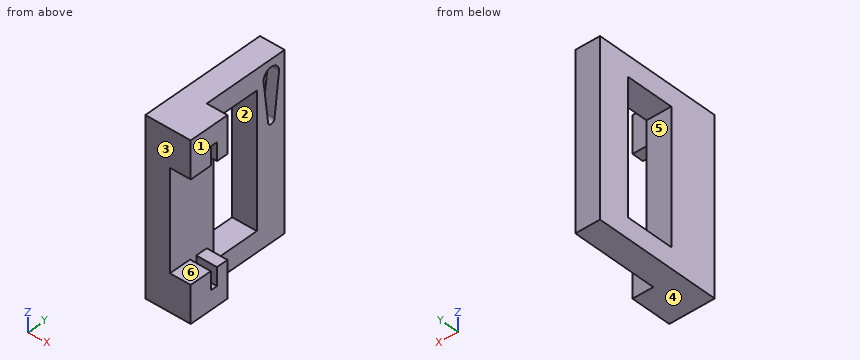
from build123d import *

# Parameters (mm, degrees)
BOSS_EXTRUDE1_DEPTH = 9
SKETCH2_W           = 8.4
SKETCH2_H           = 40.5
CUT_EXTRUDE1_DEPTH  = 40.4
SKETCH3_W           = 18.4
SKETCH3_H           = 70.5
BOSS_EXTRUDE2_DEPTH = 42.5
CUT_EXTRUDE2_DEPTH  = 8.4
SKETCH5_W           = 70.5
SKETCH5_H           = 35
CUT_EXTRUDE3_DEPTH  = 8.4
CUT_EXTRUDE4_DEPTH  = 4.6
SKETCH8_W           = 54
SKETCH8_H           = 19.4972
CUT_EXTRUDE5_DEPTH  = 11


with BuildPart() as part:
    # Sketch1 → Boss-Extrude1 (new body)
    with BuildSketch(Plane(origin=(0, 0, 0), x_dir=(1, 0, 0), z_dir=(0, 1, 0))):
        Polygon((8.4, -15), (8.4, 0), (8.4, 40.5), (8.4, 55.5), (-10, 55.5), (-10, -15), align=None)
    extrude(amount=BOSS_EXTRUDE1_DEPTH)

    # Sketch2 → Cut-Extrude1 (cut)
    with BuildSketch(Plane(origin=(0, 9, 0), x_dir=(1, 0, 0), z_dir=(0, 1, 0))):
        with Locations((4.2, 20.25)):
            Rectangle(SKETCH2_W, SKETCH2_H)
    extrude(amount=-CUT_EXTRUDE1_DEPTH, mode=Mode.SUBTRACT)

    # Sketch3 → Boss-Extrude2 (add)
    with BuildSketch(Plane(origin=(0, 9, 0), x_dir=(1, 0, 0), z_dir=(0, 1, 0))):
        with Locations((-0.8, 20.25)):
            Rectangle(SKETCH3_W, SKETCH3_H)
    extrude(amount=BOSS_EXTRUDE2_DEPTH)

    # Sketch4 → Cut-Extrude2 (cut)
    with BuildSketch(Plane(origin=(8.4, 0, 0), x_dir=(0, 0, -1), z_dir=(1, 0, 0))):
        Polygon((-0.09, 11.8), (-0.09, 44.4), (40.59, 44.4), (40.59, 11.8), (47.9, 11.8), (47.9, 9), (-7.4, 9), (-7.4, 11.8), align=None)
    extrude(amount=-CUT_EXTRUDE2_DEPTH, mode=Mode.SUBTRACT)

    # Sketch5 → Cut-Extrude3 (cut)
    with BuildSketch(Plane(origin=(8.4, 0, 0), x_dir=(0, 0, -1), z_dir=(1, 0, 0))):
        with Locations((20.25, 34)):
            Rectangle(SKETCH5_W, SKETCH5_H)
    extrude(amount=-CUT_EXTRUDE3_DEPTH, mode=Mode.SUBTRACT)

    # Sketch7 → Cut-Extrude4 (cut)
    with BuildSketch(Plane(origin=(0, 0, 0), x_dir=(0, 0, -1), z_dir=(1, 0, 0))):
        with BuildLine():
            Line((-8.5, 49.0028), (8.5259, 46.9454))
            ThreePointArc((8.5259, 46.9454), (9.9713, 45.5), (8.5259, 44.0546))
            Line((8.5259, 44.0546), (-8.5, 41.9972))
            ThreePointArc((-8.5, 41.9972), (-12.0028, 45.5), (-8.5, 49.0028))
        make_face()
    extrude(amount=-CUT_EXTRUDE4_DEPTH, mode=Mode.SUBTRACT)

    # Sketch8 → Cut-Extrude5 (cut, through all)
    with BuildSketch(Plane(origin=(0, 0, 0), x_dir=(0, 0, -1), z_dir=(1, 0, 0))):
        with Locations((20.25, 29.2486)):
            Rectangle(SKETCH8_W, SKETCH8_H)
    extrude(amount=-CUT_EXTRUDE5_DEPTH, mode=Mode.SUBTRACT)


solid = part.part
Input: part model. Units: mm. Frame: model coordinates. Face numbers are marked on the shaded views. A direction names the side the tool comes from. Coordinates: 2 decimals unless noted, no trailing zeros. Loops run counter-clockwise (first coordinate to the right, second up) from the corner with the lowest first, then second, coordinate; pieces in that order, holes last. Notation, with made-up numbers: (72, 82.5) -> (90, 82.5) arc R36 ccw to (90, 119.5) -> close; hole circle Ø6 at (-20.5, 0.25). An arc over 180 degrees is marked (long way). One line per item, written item: value.
(1) Set-up query: the marked faces 4, 5 and 6. Return all of +Z, -Z, +X, -X, +Y, -Y with unobstructed straight access to the full face (end or side cutting, diameter ignored); none if empty.
Answer below:
face 4: -Z, +X, -X, +Y, -Y
face 5: +X, -X
face 6: +X, +Y, -Y
(2) Cut plane B-B (x = -0.75). Output: boundary loops of the cut face in (y, z), then the cut area to 3 significant figures.
Answer below:
outline: (0, -55.5) -> (51.5, -55.5) -> (51.5, 15) -> (0, 15) -> close; hole (19.5, -47.25) -> (39, -47.25) -> (39, 6.75) -> (19.5, 6.75) -> close; hole (42, 8.5) -> (44.05, -8.53) arc R1.45 ccw to (46.95, -8.53) -> (49, 8.5) arc R3.5 ccw to start
area: 2,470 mm2
(3) Cut plane C-C (y = 45.5). Output: boundary loops of the cut face in (x, z), then the cut area to 3 significant figures.
Answer below:
outline: (-10, -55.5) -> (0, -55.5) -> (0, -9.97) -> (-4.6, -9.97) -> (-4.6, 12) -> (0, 12) -> (0, 15) -> (-10, 15) -> close
area: 604 mm2
(4) Draft query along Y for the marked faces 1, 2 and 3. Return one class per face: pulls with the +Y half, pulls with the -Y half, needs draft (parallel to the pull), parting line crosses it, or undercut.
Answer below:
face 1: needs draft
face 2: undercut
face 3: pulls with the -Y half
(5) Cut plane D-D (x = 5.25). Output: boundary loops of the cut face in (y, z), then the cut area to 3 significant figures.
Answer below:
outline: (0, -55.5) -> (16.5, -55.5) -> (16.5, -40.59) -> (11.8, -40.59) -> (11.8, -47.9) -> (9, -47.9) -> (9, -40.5) -> (0, -40.5) -> close; (0, 0) -> (9, 0) -> (9, 7.4) -> (11.8, 7.4) -> (11.8, 0.09) -> (16.5, 0.09) -> (16.5, 15) -> (0, 15) -> close
area: 453 mm2
(6) Cut plane A-A (z = -41.5). Output: boundary loops of the cut face in (x, y), then the cut area to 3 significant figures.
Answer below:
outline: (-10, 0) -> (8.4, 0) -> (8.4, 9) -> (0, 9) -> (0, 11.8) -> (8.4, 11.8) -> (8.4, 16.5) -> (0, 16.5) -> (0, 19.5) -> (-10, 19.5) -> close; (-10, 39) -> (0, 39) -> (0, 51.5) -> (-10, 51.5) -> close
area: 435 mm2
(7) Pin query (flat end, axial travel): pin 1 Ø2 at (x, z) = (4, 5) entering from +Y; pin 2 Ø8 at (y, z) = (36, -41) entering from +X. Return the tip coordinate at first contact, or that it passes through.
Answer below:
pin 1: stops at y = 16.5
pin 2: stops at x = 0
(8) Ray query, line 1 along Y through (x, z) = (-8, -12); line 2 along Y through (x, z) = (-1.25, 8.5); line 3 along Z through (x, y) = (-0.75, 24.5). Return the intervals inside material, ascending.
Answer below:
line 1: y = 0 to 19.5, 39 to 51.5
line 2: y = 0 to 42, 49 to 51.5
line 3: z = -55.5 to -47.25, 6.75 to 15
